For this review, take the finished solid that the model builds, in its own axes (mm). A direction names the side the tool comes from. Coordinates: 2 decimals unless noted, no trailing zeros. Loops run counter-clockwise (first coordinate to the right, second up) from the corner with the lowest first, then second, coordinate; pieces in that order, holes last. Notation, with made-up numbers: (-10.5, 25.5) -> (3.5, 25.5) arc R21 ccw to (3.5, 43.5) -> close; hole circle Ø1 at (28, -32). An arc over 180 degrees is marked (long way). Use a Markdown table: item, result.
from build123d import *

# Parameters (mm, degrees)
BOSS_EXTRUDE1_DEPTH = 8
SKETCH2_R           = 1.75
CUT_EXTRUDE1_DEPTH  = 62.359595827
CUT_EXTRUDE2_DEPTH  = 66.878676368
CUT_EXTRUDE3_DEPTH  = 3
FILLET1_R           = 2


with BuildPart() as part:
    # Sketch1 → Boss-Extrude1 (new body)
    with BuildSketch(Plane(origin=(0, 0, 0), x_dir=(1, 0, 0), z_dir=(0, 1, 0))):
        Polygon((0, 26), (0, 0), (60, 0), (60, 10), (5, 10), (5, 26), align=None)
    extrude(amount=BOSS_EXTRUDE1_DEPTH)

    # Sketch2 → Cut-Extrude1 (cut, through all)
    with BuildSketch(Plane(origin=(5, 0, 0), x_dir=(0, 0, -1), z_dir=(1, 0, 0))):
        with Locations((21.25, 4)):
            Circle(SKETCH2_R)
        with Locations((14.75, 4)):
            Circle(SKETCH2_R)
    extrude(amount=-CUT_EXTRUDE1_DEPTH, mode=Mode.SUBTRACT)

    # Sketch3 → Cut-Extrude2 (cut, through all)
    with BuildSketch(Plane(origin=(0, 8, 0), x_dir=(1, 0, 0), z_dir=(0, 1, 0))):
        with BuildLine():
            Line((10, 6.6), (55, 6.6))
            ThreePointArc((55, 6.6), (56.6, 5), (55, 3.4))
            Line((55, 3.4), (10, 3.4))
            ThreePointArc((10, 3.4), (8.4, 5), (10, 6.6))
        make_face()
    extrude(amount=-CUT_EXTRUDE2_DEPTH, mode=Mode.SUBTRACT)

    # Sketch4 → Cut-Extrude3 (cut)
    with BuildSketch(Plane.XZ):
        with BuildLine():
            Line((55, -7.85), (10, -7.85))
            ThreePointArc((10, -7.85), (7.15, -5), (10, -2.15))
            Line((10, -2.15), (55, -2.15))
            ThreePointArc((55, -2.15), (57.85, -5), (55, -7.85))
        make_face()
    extrude(amount=-CUT_EXTRUDE3_DEPTH, mode=Mode.SUBTRACT)

    # Fillet1
    fillet1_edges = [part.edges().sort_by_distance(p)[0] for p in [
        (60, 4, -10),
        (60, 4, 0),
        (0, 4, 0),
        (0, 4, -26),
    ]]
    fillet(fillet1_edges, radius=FILLET1_R)


solid = part.part
(1) Mouldability with a two-part tool opening along X and no side actions: class faces 1 (the face through (56.6, 5.5, -5)), 2 (the face through (0, 3, -13)), 3 (the face through (2.54, 4.08, -19.5)) as pulls with the +X half, pulls with the -X half, needs draft (parallel to the pull), parting line crosses it, or undercut.
Found:
| item | result |
|---|---|
| face 1 | undercut |
| face 2 | pulls with the -X half |
| face 3 | needs draft |
(2) For faces 4 (the face through (8.4, 5.5, -5)), 5 (the face through (7.15, 1.48, -5.06)), 6 (the face through (5, 4, -18)), 7 (the face through (4, 4, -26)), 8 (the face through (59.4, 4.06, -0.57)), list the 3-axis set-ups (+Z, -Z, +X, -X, +Y, -Y) from which the entire face can be reached by the end or side of a thin tool; tool diameter is ignored.
Found:
| item | result |
|---|---|
| face 4 | +Y, -Y |
| face 5 | -Y |
| face 6 | -Z, +X, +Y, -Y |
| face 7 | -Z, +X, -X, +Y, -Y |
| face 8 | +Z, +X, +Y, -Y |
(3) For line 1 along Z through (x, y) = (54.5, 6.5); line 2 along Y through (x, z) = (3.95, -21.25); line 3 along X through (y, z) = (6, -22), list the stretches that pass through material, from the lowest coordinate up.
Found:
| item | result |
|---|---|
| line 1 | z = -10 to -6.6, -3.4 to 0 |
| line 2 | y = 0 to 2.25, 5.75 to 8 |
| line 3 | x = 0 to 5 |
(4) Take a section at B-B on z = -5. Write out the cut boundary in (x, y).
Found:
| item | result |
|---|---|
| outline | (0, 0) -> (7.15, 0) -> (7.15, 3) -> (8.4, 3) -> (8.4, 8) -> (0, 8) -> close; (56.6, 3) -> (57.85, 3) -> (57.85, 0) -> (60, 0) -> (60, 8) -> (56.6, 8) -> close |
(5) For pin 1 Ø2 at (x, y) = (20, 6) entering from -Z; pin 2 Ø2 at (y, z) = (4, -14.75) entering from +X (1 decimal); pin 3 Ø2.5 at (y, z) = (2, -14.5) entering from +X, all flat-tipped, find the tip position at first contact; note any pin that passes through.
Found:
| item | result |
|---|---|
| pin 1 | stops at z = -10 |
| pin 2 | passes through |
| pin 3 | stops at x = 5 |
(6) Take a section at A-A on y = 4. Write out the cut boundary in (x, z), plus the area to 3 significant figures.
Found:
| item | result |
|---|---|
| outline | (0, -24) arc R2 ccw to (2, -26) -> (5, -26) -> (5, -23) -> (0, -23) -> close; (0, -19.5) -> (5, -19.5) -> (5, -16.5) -> (0, -16.5) -> close; (0, -13) -> (5, -13) -> (5, -10) -> (58, -10) arc R2 ccw to (60, -8) -> (60, -2) arc R2 ccw to (58, 0) -> (2, 0) arc R2 ccw to (0, -2) -> close; hole (10, -6.6) -> (55, -6.6) arc R1.6 ccw to (55, -3.4) -> (10, -3.4) arc R1.6 ccw to start |
| area | 490 mm^2 |
(7) Take a section at D-D on y = 7.25. Write out the cut boundary in (x, z), plus the area to 3 significant figures.
Found:
| item | result |
|---|---|
| outline | (0, -24) arc R2 ccw to (2, -26) -> (5, -26) -> (5, -10) -> (58, -10) arc R2 ccw to (60, -8) -> (60, -2) arc R2 ccw to (58, 0) -> (2, 0) arc R2 ccw to (0, -2) -> close; hole (10, -6.6) -> (55, -6.6) arc R1.6 ccw to (55, -3.4) -> (10, -3.4) arc R1.6 ccw to start |
| area | 525 mm^2 |
(8) Take a section at C-C on x = 42.5. Write out the cut boundary in (y, z).
Found:
| item | result |
|---|---|
| outline | (0, -10) -> (8, -10) -> (8, -6.6) -> (3, -6.6) -> (3, -7.85) -> (0, -7.85) -> close; (0, -2.15) -> (3, -2.15) -> (3, -3.4) -> (8, -3.4) -> (8, 0) -> (0, 0) -> close |
